```python
from build123d import *

# Parameters (mm, degrees)
SKETCH1_W                   = 622.3
SKETCH1_H                   = 76.2
BOSS_EXTRUDE1_DEPTH         = 6.35
F_1_4_0_25_DIAMETER_HOLE1_D = 6.35
LPATTERN1_COUNT             = 4
LPATTERN1_PITCH             = 114.3
SKETCH4_R                   = 19.05
BOSS_EXTRUDE3_DEPTH         = 6.35


with BuildPart() as part:
    # Sketch1 → Boss-Extrude1 (new body)
    with BuildSketch(Plane.XY.offset(457.2)):
        with Locations((0, 571.5)):
            Rectangle(SKETCH1_W, SKETCH1_H)
    extrude(amount=BOSS_EXTRUDE1_DEPTH)

    # 1/4 (0.25) Diameter Hole1 (through all)
    with Locations(Plane.XY.offset(463.55)):
        with Locations((171.45, 577.85)):
            f_1_4_0_25_diameter_hole1 = Hole(F_1_4_0_25_DIAMETER_HOLE1_D / 2)

    # LPattern1: 1/4 (0.25) Diameter Hole1 ×4
    with Locations(*[(-i * LPATTERN1_PITCH, 0, 0) for i in range(1, LPATTERN1_COUNT)]):
        add(f_1_4_0_25_diameter_hole1, mode=Mode.SUBTRACT)

    # Sketch4 → Boss-Extrude3 (add)
    with BuildSketch(Plane.XY.offset(463.55)):
        with BuildLine():
            Line((311.15, 533.4), (372.587826171, 546.832705994))
            ThreePointArc((372.587826171, 546.832705994), (397.37252749, 581.26052894), (365.806235462, 609.6))
            Line((365.806235462, 609.6), (311.15, 609.6))
            Line((311.15, 609.6), (311.15, 533.4))
        make_face()
        with Locations((365.806235462, 577.85)):
            Circle(SKETCH4_R, mode=Mode.SUBTRACT)
    boss_extrude3 = extrude(amount=-BOSS_EXTRUDE3_DEPTH)

    # Mirror1: Boss-Extrude3 across plane
    add(boss_extrude3.mirror(Plane(origin=(0, 0, 0), x_dir=(0, 0, 1), z_dir=(1, 0, 0))))


solid = part.part
```
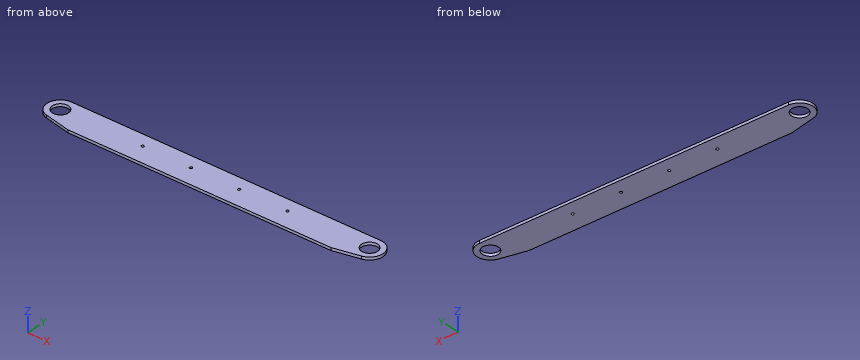
Work out the finished part from the listing and answer in its coordinate system (mm). Coordinates: 2 decimals unless noted, no trailing zeros. Write each loop counter-clockwise with the first axis right and the second up, starting at its lowest first coordinate (ties: lowest second). Pieces come first, ordered by that corner, then holes.
Q1. Find the intervals of material crossed by line 1 (Y direction, x = 171.45, z = 459) (3 decimals); line 2 (X direction, y = 564.5, z = 461.5); line 3 (X direction, y = 584.5, z = 462), in increasing order.
Q2. A cutting plane is placed at A-A, the plane z = 458.25. Give the vertices of the cut face in (x, y) (3 decimals), then the cut area to 3 significant figures.
Q3. Each of these flat-tipped pins is pushed along its axis until it touches: pin 1 Ø1 at (y, z) = (590.5, 460.5) entering from +X; pin 2 Ø1.5 at (y, z) = (581, 458) entering from +X. Where does it stop, or does it pass through?
Q4. A cutting plane is placed at B-B, the plane y = 566. Give the vertices of the cut face in (x, z), then the cut area to 3 significant figures.
Findings below:
1. line 1: y = 533.4 to 574.675, 581.025 to 609.6
1. line 2: x = -394.61 to -379.4, -352.22 to 352.22, 379.4 to 394.61
1. line 3: x = -396.85 to -383.66, -347.95 to 347.95, 383.66 to 396.85
2. outline: (-372.588, 546.833) - (-311.15, 533.4) - (311.15, 533.4) - (372.588, 546.833) arc R31.75 ccw to (365.806, 609.6) - (-365.806, 609.6) arc R31.75 ccw to start; hole circle Ø38.1 at (-365.806, 577.85); hole circle Ø6.35 at (-171.45, 577.85); hole circle Ø6.35 at (-57.15, 577.85); hole circle Ø6.35 at (57.15, 577.85); hole circle Ø6.35 at (171.45, 577.85); hole circle Ø38.1 at (365.806, 577.85)
2. area: 55,900 mm2
3. pin 1: stops at x = 395.14
3. pin 2: stops at x = 397.47
4. outline: (-395.26, 457.2) - (-380.72, 457.2) - (-380.72, 463.55) - (-395.26, 463.55) - close; (-350.89, 457.2) - (350.89, 457.2) - (350.89, 463.55) - (-350.89, 463.55) - close; (380.72, 457.2) - (395.26, 457.2) - (395.26, 463.55) - (380.72, 463.55) - close
4. area: 4,640 mm2
